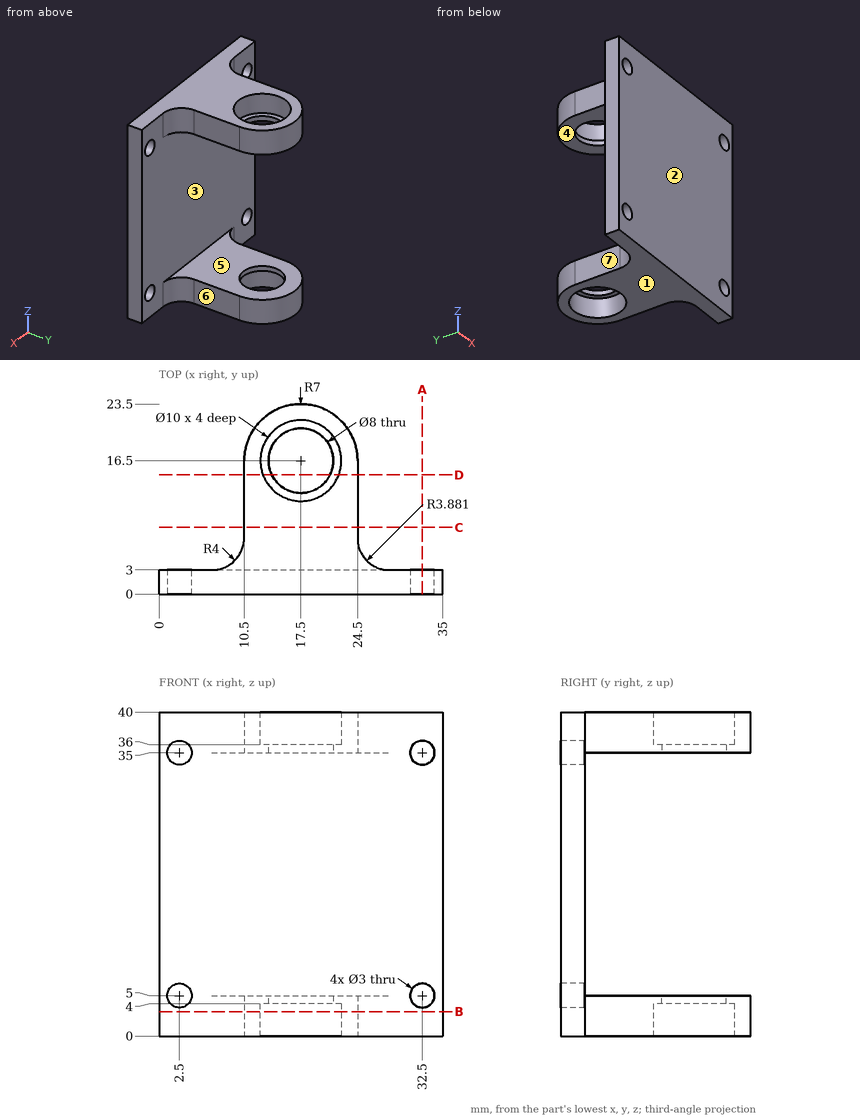
Check sheet for the drawn part. Datum: minimum x, y, z corner. Units: mm. A direction names the side the tool comes from. Coordinates: 2 decimals unless noted, no trailing zeros. Order: outer loops, then holes, each group sorted by start corner. A loop starts at its lowest first (then second) coordinate and runs counter-clockwise, first axis right, second up. Notation, with made-up numbers: M -15,30 L 34,30 A29 ccw 34,52 Z; hole C 12.5,85.25 d10. An arc over 180 degrees is marked long. One line per question, with ' | ' between items. Start each with the question number.
Item 1: Material ranges on line 1 (Z direction, x = 32.5, y = 0.9); line 2 (Z direction, x = 23, y = 11.5); line 3 (Y direction, x = 17.5, z = 4.4), recorded low to high.
Item 2: Sectioned sample at B-B on z = 3. Record the cut outline in (x, y).
Item 3: Sectioned sample at C-C on y = 8.25. Record the cut outline in (x, z), and give its area (3 significant figures).
Item 4: Gauge pin test, flat ends, axial feed: P1, Ø12, axis at x = 27.5, z = 27.5, coming from the +Y side; P2, Ø5.5, axis at y = 13, z = 2, coming from the +X side; P3, Ø9, axis at x = 17.5, y = 16.5, coming from the -Z side. Record the tip position at first contact, or that the pin passes through.
Item 5: Access from +Z, -Z, +X, -X, +Y, -Y to the whole of each face (thin tool, end or side, straight path). Record for the marked faces 5, 6 and 7.
Item 6: Sectioned sample at A-A on x = 32.5. Record the cut outline in (y, z).
Item 7: Sectioned sample at D-D on y = 14.75. Record the cut outline in (x, z), and give its area (3 significant figures).
Item 8: Mould release check, pull along Z, two halves, no side actions. Record for the marked faces 1, 2, 3 and 4: pulls with the +Z half, pulls with the -Z half, needs draft (parallel to the pull), parting line crosses it, or undercut.
Answer below:
1) line 1: z = 0 to 3.5, 6.5 to 33.5, 36.5 to 40 | line 2: z = 0 to 5, 35 to 40 | line 3: y = 0 to 12.5, 20.5 to 23.5
2) outline: M 0,0 L 35,0 L 35,3 L 28.38,3 A3.88 cw 24.5,6.88 L 24.5,16.5 A7 ccw 10.5,16.5 L 10.5,7 A4 cw 6.5,3 L 0,3 Z; hole C 17.5,16.5 d10
3) outline: M 10.5,0 L 24.5,0 L 24.5,5 L 10.5,5 Z; M 10.5,35 L 24.5,35 L 24.5,40 L 10.5,40 Z | area: 140 mm^2
4) P1: stops at y = 3 | P2: stops at x = 24.5 | P3: stops at z = 4
5) face 5: +X, -X, +Y | face 6: +Z, -Z, +X, +Y | face 7: +Z, -Z, -X, +Y
6) outline: M 0,0 L 3,0 L 3,3.5 L 0,3.5 Z; M 0,6.5 L 3,6.5 L 3,33.5 L 0,33.5 Z; M 0,36.5 L 3,36.5 L 3,40 L 0,40 Z
7) outline: M 10.5,0 L 12.82,0 L 12.82,4 L 13.9,4 L 13.9,5 L 10.5,5 Z; M 10.5,35 L 13.9,35 L 13.9,36 L 12.82,36 L 12.82,40 L 10.5,40 Z; M 21.1,4 L 22.18,4 L 22.18,0 L 24.5,0 L 24.5,5 L 21.1,5 Z; M 21.1,35 L 24.5,35 L 24.5,40 L 22.18,40 L 22.18,36 L 21.1,36 Z | area: 50.7 mm^2
8) face 1: pulls with the -Z half | face 2: needs draft | face 3: undercut | face 4: undercut
